Answer from the drawing. Dimensions are ordinates in mm from the lowest x, y and z of the part. A direction names the side the tool comes from. Give positions to 0.01 mm unless a question says otherwise; leave off trailing zeros. Write each loop counter-clockwise with the first axis right and the second up, starting at its lowest first coordinate (ties: lowest second). Pieces come first, ordered by that corner, then holes.
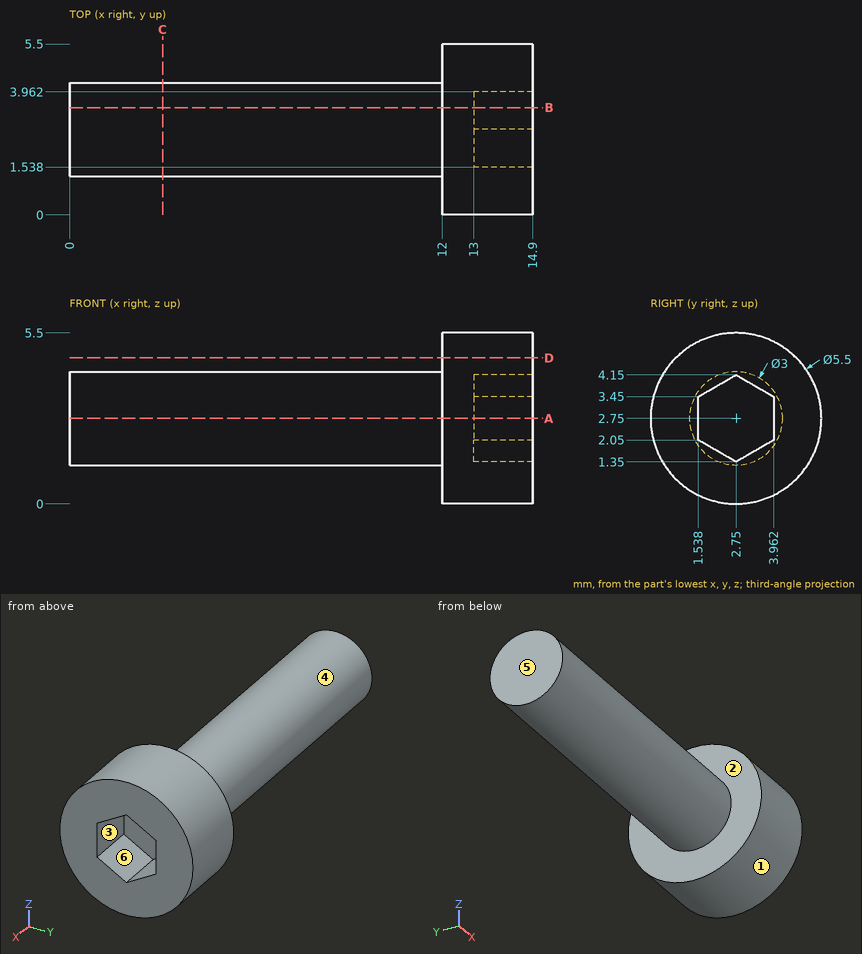
Item 1: Determine the mould class of the marked faces 1, 2 and 3 for opening direction Z: pulls with the +Z half, pulls with the -Z half, needs draft (parallel to the pull), parting line crosses it, or undercut.
Conclusion:
face 1: parting line crosses it
face 2: needs draft
face 3: undercut
Item 2: A cutting plane is placed at C-C, the plane x = 3. Give the vertices of the cut face in (y, z).
Conclusion:
outline: circle Ø3 at (2.75, 2.75)
Item 3: A cutting plane is placed at D-D, the plane z = 4.7. Give the vertices of the cut face in (x, y).
Conclusion:
outline: (12, 0.81) - (14.9, 0.81) - (14.9, 4.69) - (12, 4.69) - close
Item 4: A cutting plane is placed at A-A, the plane z = 2.75. Give the vertices of the cut face in (x, y).
Conclusion:
outline: (0, 1.25) - (12, 1.25) - (12, 0) - (14.9, 0) - (14.9, 1.54) - (13, 1.54) - (13, 3.96) - (14.9, 3.96) - (14.9, 5.5) - (12, 5.5) - (12, 4.25) - (0, 4.25) - close
Item 5: Which of the six approach directions +Z, -Z, +X, -X, +Y, -Y give full straight-line access (tool end or side, diameter ignored) to the marked faces 4, 5 and 6?
Conclusion:
face 4: -X
face 5: +Z, -Z, -X, +Y, -Y
face 6: +X
Item 6: Each of these flat-tipped pins is pushed along its axis until it touches: P1, Ø2, axis at x = 2, z = 1.5, coming from the +Y side; P2, Ø1.5, axis at x = 11.5, y = 4.5, coming from the +Z side; P3, Ø0.7, axis at y = 3.5, z = 3, coming from the +X side. Where does it stop, or does it pass through?
Conclusion:
P1: stops at y = 4.23
P2: stops at z = 5.23
P3: stops at x = 13
Item 7: A cutting plane is placed at B-B, the plane y = 3.45. Give the vertices of the cut face in (x, z).
Conclusion:
outline: (0, 1.42) - (12, 1.42) - (12, 0.09) - (14.9, 0.09) - (14.9, 1.75) - (13, 1.75) - (13, 3.75) - (14.9, 3.75) - (14.9, 5.41) - (12, 5.41) - (12, 4.08) - (0, 4.08) - close
Item 8: Consider probe 1 along X at (y, z) = (3.15, 4.8); probe 2 along Z at (x, y) = (1.5, 2.8); probe 3 along Z at (x, y) = (14, 3.7). Determine where each line is inside the solid, lowest interval first.
Conclusion:
probe 1: x = 12 to 14.9
probe 2: z = 1.25 to 4.25
probe 3: z = 0.17 to 1.9, 3.6 to 5.33
